```python
from build123d import *

# Parameters (mm, degrees)
SCHIZZO1_R                   = 0.458996056
ESTRUSIONE_ESTRUSIONE1_DEPTH = 0.6


with BuildPart() as part:
    # Schizzo1 → Estrusione-Estrusione1 (new body)
    with BuildSketch(Plane.XZ.offset(0.3)):
        with BuildLine():
            Line((-2.34, 5.13), (-2.34, 3.993043952))
            ThreePointArc((-2.34, 3.993043952), (-2.395647685, 3.763803858), (-2.550204082, 3.585590487))
            ThreePointArc((-2.550204082, 3.585590487), (-3.12270208, 3.099795432), (-3.604268995, 2.52373632))
            add(Edge.make_bspline(
                [(-3.604268995, 2.52373632), (-3.853924568, 2.156927576), (-4.029511845, 1.735833882), (-4.145169154, 1.307464944), (-4.308172181, 0.703737997), (-4.360675474, 0.06363484), (-4.320124497, -0.560393871), (-4.278553695, -1.200116418), (-4.137438556, -1.845937547), (-3.877676401, -2.432023456), (-3.723583884, -2.779693241), (-3.52331205, -3.113059535), (-3.273444303, -3.39973861), (-3.112104376, -3.58484766), (-2.9274837, -3.75281032), (-2.724488073, -3.89097221)],
                knots=[0, 0, 0, 0, 0.001331123, 0.001331123, 0.001331123, 0.003211952, 0.003211952, 0.003211952, 0.005142922, 0.005142922, 0.005142922, 0.006280106, 0.006280106, 0.006280106, 0.007010759, 0.007010759, 0.007010759, 0.007010759], degree=3))
            ThreePointArc((-2.724488073, -3.89097221), (0, -4.75), (2.724488073, -3.89097221))
            add(Edge.make_bspline(
                [(2.724488073, -3.89097221), (3.02256608, -3.682255743), (3.280103619, -3.409405395), (3.48806342, -3.110798992), (3.7651858, -2.712883068), (3.966732048, -2.257894847), (4.103489225, -1.792672996), (4.28909221, -1.161287017), (4.363995711, -0.488820559), (4.33114693, 0.168459959), (4.304204363, 0.707561374), (4.203554262, 1.252009555), (4.008527428, 1.755319372), (3.903955576, 2.02519013), (3.770275035, 2.286655125), (3.604268995, 2.52373632)],
                knots=[0, 0, 0, 0, 0.001091658, 0.001091658, 0.001091658, 0.002547666, 0.002547666, 0.002547666, 0.004529951, 0.004529951, 0.004529951, 0.006151973, 0.006151973, 0.006151973, 0.007014946, 0.007014946, 0.007014946, 0.007014946], degree=3))
            ThreePointArc((3.604268995, 2.52373632), (3.12270208, 3.099795432), (2.550204082, 3.585590487))
            ThreePointArc((2.550204082, 3.585590487), (2.395647685, 3.763803858), (2.34, 3.993043952))
            Line((2.34, 3.993043952), (2.34, 5.13))
            ThreePointArc((2.34, 5.13), (2.24890321, 5.417746703), (2.008807339, 5.600642202))
            ThreePointArc((2.008807339, 5.600642202), (1.480262865, 5.762926501), (0.938936535, 5.875448764))
            ThreePointArc((0.938936535, 5.875448764), (0.842129544, 5.848255068), (0.8, 5.756952319))
            Line((0.8, 5.756952319), (0.8, 3.759055732))
            ThreePointArc((0.8, 3.759055732), (0.825598581, 3.684972184), (0.891472868, 3.642495865))
            ThreePointArc((0.891472868, 3.642495865), (0, -3.75), (-0.891472868, 3.642495865))
            ThreePointArc((-0.891472868, 3.642495865), (-0.825598581, 3.684972184), (-0.8, 3.759055732))
            Line((-0.8, 3.759055732), (-0.8, 5.756952319))
            ThreePointArc((-0.8, 5.756952319), (-0.842129544, 5.848255068), (-0.938936535, 5.875448764))
            ThreePointArc((-0.938936535, 5.875448764), (-1.480262865, 5.762926501), (-2.008807339, 5.600642202))
            ThreePointArc((-2.008807339, 5.600642202), (-2.24890321, 5.417746703), (-2.34, 5.13))
        make_face()
        with Locations((1.57, 4.598363042)):
            Circle(SCHIZZO1_R, mode=Mode.SUBTRACT)
        with Locations((-1.57, 4.598363042)):
            Circle(SCHIZZO1_R, mode=Mode.SUBTRACT)
    extrude(amount=-ESTRUSIONE_ESTRUSIONE1_DEPTH)


solid = part.part
```
Design review of the part built by this model. Coordinates are the model's own, in mm. Round coordinates to 2 decimals unless told otherwise and drop trailing zeros. Order: outer loops, then holes, each group sorted by start corner. A loop starts at its lowest first (then second) coordinate and runs counter-clockwise, first axis right, second up. Notation, with made-up numbers: (-38.5, -3) - (-33.5, -3) arc R23 cw to (-33.5, 10) - close; hole circle Ø7 at (-38.75, 7.5). An arc over 180 degrees is marked (long way). One line per question, with ' | ' between items.
Item 1: Wall thickness on line 1 (Z direction, x = -1.57, y = 0.1); line 2 (X direction, y = -0.15, z = 3.75); line 3 (X direction, y = -0.1, z = 4): over which ranges is each line inside the solid? List them lowest first. Write a range as [from, to].
Checks:
line 1: [-4.48, -3.41], [3.41, 4.14], [5.06, 5.74] | line 2: [-2.4, -0.8], [0.8, 2.4] | line 3: [-2.34, -0.8], [0.8, 2.34]
Item 2: Take a section at A-A, the plane x = -1.5. Write out the cut boundary in (y, z), then the cut area to 3 significant figures.
Checks:
outline: (-0.3, -4.51) - (0.3, -4.51) - (0.3, -3.44) - (-0.3, -3.44) - close; (-0.3, 3.44) - (0.3, 3.44) - (0.3, 4.14) - (-0.3, 4.14) - close; (-0.3, 5.05) - (0.3, 5.05) - (0.3, 5.76) - (-0.3, 5.76) - close | area: 1.49 mm²
Item 3: Take a section at D-D, the plane y = 0.05. Give the number of separate pieces and of enclosed holes in the cut face, then the cut area to 3 significant figures.
Checks:
separate pieces: 1 | enclosed holes: 2 | area: 22.2 mm²
Item 4: Draft analysis for pull direction Z (two halves, no side actions). For faces 1 (the face through (-0.04, 0, -4.75)), 2 (the face through (1.994, -0.004, 4.423)), 3 (the face through (4, 0.3, 1)), state which applies: +Z half, -Z half, draft (parallel to the pull), parting line (faces both ways), or undercut.
Checks:
face 1: -Z half | face 2: undercut | face 3: draft
Item 5: Take a section at B-B, the plane z = 2.75. Write out the cut boundary in (x, y).
Checks:
outline: (-3.43, -0.3) - (-2.55, -0.3) - (-2.55, 0.3) - (-3.43, 0.3) - close; (2.55, -0.3) - (3.43, -0.3) - (3.43, 0.3) - (2.55, 0.3) - close
Item 6: Take a section at C-C, the plane x = 0. Write out the cut boundary in (y, z).
Checks:
outline: (-0.3, -4.75) - (0.3, -4.75) - (0.3, -3.75) - (-0.3, -3.75) - close
